Build history of the part. All positions in model axes, mm. A direction names the side the tool comes from. Coordinates: 2 decimals unless noted, no trailing zeros. Order: outer loops, then holes, each group sorted by start corner. A loop starts at its lowest first (then second) coordinate and runs counter-clockwise, first axis right, second up. Notation, with made-up numbers: (79, -26) - (120, -26) arc R35 cw to (120, 10) - close; hole circle Ø1 at (-39, 9.5). An arc over 180 degrees is marked (long way). Return JSON: item names as keys, results as strings.
Autodesk Inventor part; units mm, degrees
ref_plane "YZ Plane" through (0, 0, 0) normal (1, 0, 0) x (0, 1, 0)
ref_plane "XZ Plane" through (0, 0, 0) normal (0, 1, 0) x (-1, 0, 0)
ref_plane "XY Plane" through (0, 0, 0) normal (0, 0, 1) x (1, 0, 0)
sketch "Sketch1" plane through (0, 0, 0) normal (0, 1, 0) x (-1, 0, 0)
  line L0 (0, 0) -> (55.5625, 0)
  line L1 (55.5625, 0) -> (55.5625, -84.1375)
  line L2 (55.5625, -84.1375) -> (0, -84.1375)
  line L3 (0, -84.1375) -> (0, 0)
  line L4 (55.5625, 0) -> (0, 0)
  line L5 (0, 0) -> (0, 4.7625)
  line L6 (0, 4.7625) -> (55.5625, 4.7625)
  line L7 (55.5625, 4.7625) -> (55.5625, 0)
  line L8 (55.5625, -84.1375) -> (0, -84.1375)
  line L9 (0, -84.1375) -> (0, -88.9)
  line L10 (0, -88.9) -> (55.5625, -88.9)
  line L11 (55.5625, -88.9) -> (55.5625, -84.1375)
  line L12 (55.5625, 4.7625) -> (60.325, 4.7625)
  line L13 (55.5625, 1.7145) -> (55.5625, 4.7625)
  line L14 (55.5625, -84.1375) -> (60.325, -84.1375)
  line L15 (60.325, -84.1375) -> (60.325, -88.9)
  line L16 (60.325, -88.9) -> (55.5625, -88.9)
  line L17 (55.5625, -88.9) -> (55.5625, -84.1375)
  line L18 (0, -84.1375) -> (-4.7625, -84.1375)
  line L19 (-4.7625, -84.1375) -> (-4.7625, -88.9)
  line L20 (-4.7625, -88.9) -> (0, -88.9)
  line L21 (0, -88.9) -> (0, -84.1375)
  line L22 (0, 4.7625) -> (-4.7625, 4.7625)
  line L23 (-4.7625, 4.7625) -> (-4.7625, 1.7145)
  line L24 (0, 1.7145) -> (0, 4.7625)
  line L25 (53.1812, 3.175) -> (2.3812, 3.175)
  line L26 (2.3812, 3.175) -> (2.3812, 1.5875)
  line L27 (2.3812, 1.5875) -> (53.1812, 1.5875)
  line L28 (53.1812, 1.5875) -> (53.1812, 3.175)
  line L29 (53.975, 3.9687) -> (1.5875, 3.9687)
  line L30 (1.5875, 3.9687) -> (1.5875, 0.7938)
  line L31 (1.5875, 0.7938) -> (53.975, 0.7938)
  line L32 (53.975, 0.7938) -> (53.975, 3.9687)
  line L33 (60.325, 4.7625) -> (55.5625, 4.7625)
  line L34 (55.5625, 4.7625) -> (55.5625, 0)
  line L35 (55.5625, 0) -> (60.325, 0)
  line L36 (60.325, 0) -> (60.325, 4.7625)
  line L37 (0, 4.7625) -> (-4.7625, 4.7625)
  line L38 (-4.7625, 4.7625) -> (-4.7625, 0)
  line L39 (-4.7625, 0) -> (0, 0)
  line L40 (0, 0) -> (0, 4.7625)
  point P0 (55.5625, 2.3813)
  point P1 (0, -88.9)
  point P2 (-4.7625, 1.7145)
  dimension "d0" = 55.5625
  dimension "d1" = 84.1375
  dimension "d2" = 55.5625
  dimension "d4" = 55.5625
  dimension "d7" = 4.7625
  dimension "d8" = 4.7625
  dimension "d9" = 4.7625
  dimension "d10" = 50.8
  dimension "d12" = 1.5875
  dimension "d13" = 1.5875
  dimension "d14" = 2.3813
  dimension "d15" = 0.7937
extrude "Extrusion1" add sketch "Sketch1" along normal blind 4.7625 contours L0 L1 L2 L3
extrude "Extrusion2" add sketch "Sketch1" along normal blind 1.5875 contours L5 L6 L7 L0 | L2 L11 L10 L9 | L9 L20 L19 L18 | L14 L15 L16 L11 | L28 L27 L26 L25 | L32 L31 L30 L29
extrude "Extrusion3" add sketch "Sketch1" along normal blind 1.5875 contours L39 L38 L23 L22 L5 | L7 L12 L36 L35
extrude "Extrusion4" add sketch "Sketch1" along normal blind 3.175 contours L28 L27 L26 L25
extrude "Extrusion5" add sketch "Sketch1" against normal blind 7.9375 contours L28 L27 L26 L25 | L32 L31 L30 L29
fillet "Fillet1" radius 2.3813 8 edges at (-60.325, 0.7937, 4.7625) (-60.325, 0.7937, 0) (4.7625, 0.7937, 4.7625) (4.7625, 0.7937, 0) (4.7625, 0.7937, -84.1375) (4.7625, 0.7937, -88.9) (-60.325, 0.7937, -88.9) (-60.325, 0.7937, -84.1375)
properties part number "LCD_Display"
1. Drop flat-ended pins along their axis: pin 1 (5 mm diameter, centred on y = -1, z = -68, fed in from -X); pin 2 (2.5 mm diameter, centred on x = -30.5, y = -4, fed in from +Z); pin 3 (2.5 mm diameter, centred on y = -2, z = 2.5, fed in from -X) (3 decimals); pin 4 (1.5 mm diameter, centred on x = -53, y = 2, fed in from +Z). Give the stop position or say it passes through.
Check values:
{"pin 1": "x = -55.56", "pin 2": "z = 3.97", "pin 3": "x = -53.975", "pin 4": "z = 4.76"}
2. Probe L1, parallel to Z at x = -47.5, y = 2.25 (1 decimal); L2, parallel to Z at x = -3.5, y = -5.5; L3, parallel to X at y = 2.25, z = -48. List the from-to ranges inside material, lowest first.
Check values:
{"L1": "-84.1 to 0, 1.6 to 3.2", "L2": "0.79 to 3.97", "L3": "-55.56 to 0"}
3. Tool access for faces 1 (the cylindrical face through (4.05, 0.8, -84.82)), 2 (the flat face through (-27, 3, 0)), 3 (the flat face through (-55.562, 2, -41)): list every direction of +Z, -Z, +X, -X, +Y, -Y with a clear straight run to the whole face (end or side of a thin tool).
Check values:
{"face 1": "+X, +Y, -Y", "face 2": "+X, -X, +Y", "face 3": "-X, +Y, -Y"}
4. Cut at C-C on z = -54.5. Give the cut face in (x, y), plus the area to 3 significant figures.
Check values:
{"outline": "(-55.56, 0) - (0, 0) - (0, 4.76) - (-55.56, 4.76) - close", "area": "265 mm²"}
5. Cut at B-B on y = -4.75. Give the cut face in (x, z) (1 decimal), plus the area to 3 significant figures.
Check values:
{"outline": "(-54, 0.8) - (-1.6, 0.8) - (-1.6, 4) - (-54, 4) - close", "area": "166 mm²"}
6. Cut at A-A on x = -22.5. Give the cut face in (y, z) (1 decimal), plus the area to 3 significant figures.
Check values:
{"outline": "(-7.9, 0.8) - (0, 0.8) - (0, -88.9) - (1.6, -88.9) - (1.6, -84.1) - (4.8, -84.1) - (4.8, 0) - (1.6, 0) - (1.6, 1.6) - (3.2, 1.6) - (3.2, 3.2) - (1.6, 3.2) - (1.6, 4.8) - (0, 4.8) - (0, 4) - (-7.9, 4) - close", "area": "444 mm²"}
7. Mould opens along Z. For faces 4 (the cylindrical face through (-59.646, 0.805, -84.853)), 5 (the cylindrical face through (4.084, 0.805, -88.184)), 6 (the flat face through (-27, 1.588, -86)) say: pulls with the +Z half, pulls with the -Z half, needs draft (parallel to the pull), parting line crosses it, or undercut.
Check values:
{"face 4": "undercut", "face 5": "pulls with the -Z half", "face 6": "needs draft"}
